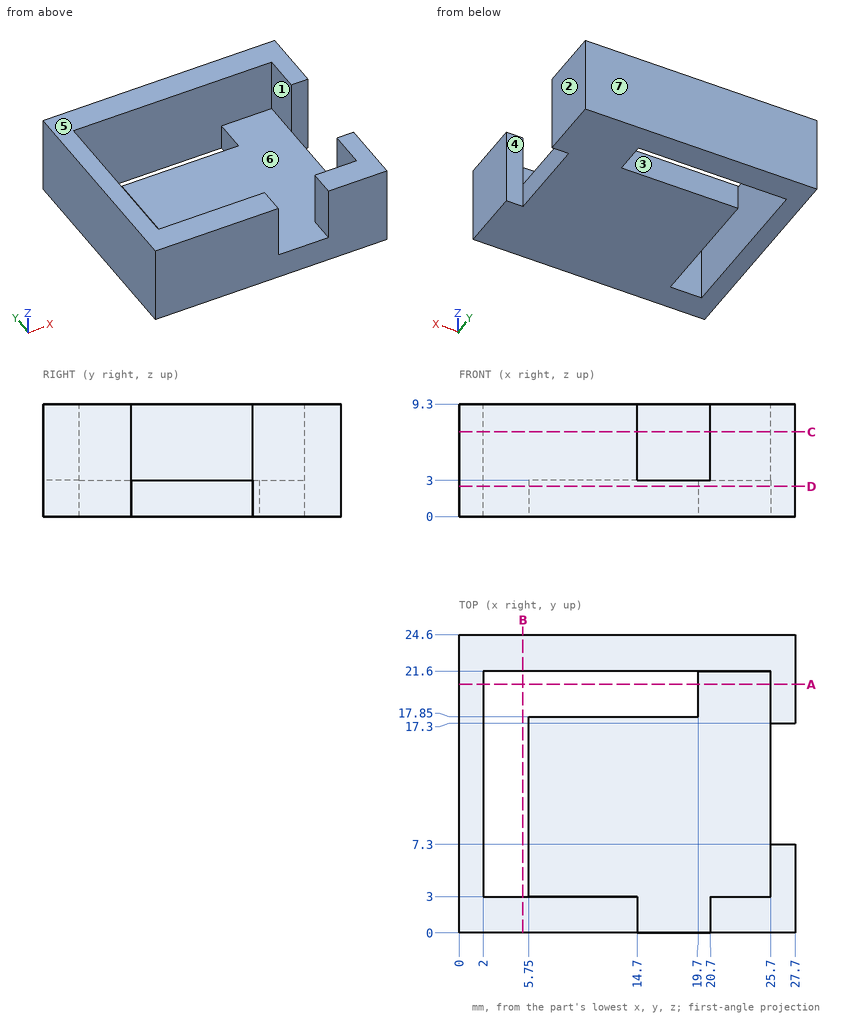
Design review of the part shown in the three views and the two pictorial views. Dimensions are in mm from the part's minimum x, y and z. A direction names the side the tool comes from. Coordinates: 2 decimals unless noted, no trailing zeros. Order: outer loops, then holes, each group sorted by start corner. A loop starts at its lowest first (then second) coordinate and runs counter-clockwise, first axis right, second up.
Item 1: Take a section at A-A, the plane y = 20.5. Write out the cut boundary in (x, z), then the cut area to 3 significant figures.
Item 2: Take a section at D-D, the plane z = 2.5. Write out the cut boundary in (x, y).
Item 3: For pin 1 Ø3.5 at (y, z) = (13.5, 2) entering from +X; pin 2 Ø8 at (x, y) = (16.5, 17.5) entering from +Z, all flat-tipped, find the tip position at first contact; note any pin that passes through.
Item 4: For line 1 (X direction, y = 5, z = 5.5); line 2 (Y direction, x = 3, z = 4); line 3 (X direction, y = 13.5, z = 0.5), list the stretches that pass through material, from the lowest coordinate up.
Item 5: For the marked faces 1, 2, 3 and 4, list the 3-axis set-ups (+Z, -Z, +X, -X, +Y, -Y) from which the entire face can be reached by the end or side of a thin tool; tool diameter is ignored.
Item 6: The part is to be moulded in two halves that separate along Y. For the marked faces 5, 6 and 7, say which applies: pulls with the +Y half, pulls with the -Y half, needs draft (parallel to the pull), parting line crosses it, or undercut.
Item 7: Take a section at C-C, the plane z = 7. Write out the cut boundary in (x, y).
Item 8: Take a section at B-B, the plane x = 5.25. Write out the cut boundary in (y, z).
The answers:
1. outline: (0, 0) - (2, 0) - (2, 9.3) - (0, 9.3) - close; (19.7, 0) - (27.7, 0) - (27.7, 9.3) - (25.7, 9.3) - (25.7, 3) - (19.7, 3) - close
1. area: 55.2 mm2
2. outline: (0, 0) - (27.7, 0) - (27.7, 7.3) - (25.7, 7.3) - (25.7, 17.3) - (27.7, 17.3) - (27.7, 24.6) - (0, 24.6) - close; hole (2, 3) - (5.75, 3) - (5.75, 17.85) - (19.7, 17.85) - (19.7, 21.6) - (2, 21.6) - close
3. pin 1: stops at x = 25.7
3. pin 2: stops at z = 3
4. line 1: x = 0 to 2, 25.7 to 27.7
4. line 2: y = 0 to 3, 21.6 to 24.6
4. line 3: x = 0 to 2, 5.75 to 25.7
5. face 1: +Z
5. face 2: +Z, -Z, +X, +Y, -Y
5. face 3: +Z, -Z
5. face 4: +Z, -Z, +X
6. face 5: needs draft
6. face 6: undercut
6. face 7: pulls with the +Y half
7. outline: (0, 0) - (14.7, 0) - (14.7, 3) - (2, 3) - (2, 21.6) - (25.7, 21.6) - (25.7, 17.3) - (27.7, 17.3) - (27.7, 24.6) - (0, 24.6) - close; (20.7, 0) - (27.7, 0) - (27.7, 7.3) - (25.7, 7.3) - (25.7, 3) - (20.7, 3) - close
8. outline: (0, 0) - (3, 0) - (3, 9.3) - (0, 9.3) - close; (21.6, 0) - (24.6, 0) - (24.6, 9.3) - (21.6, 9.3) - close
